For this review, take the finished solid that the model builds, in its own axes (mm). Face numbers are marked on the shaded views. A direction names the side the tool comes from. Coordinates: 2 decimals unless noted, no trailing zeros. Order: outer loops, then holes, each group sorted by start corner. A loop starts at its lowest first (then second) coordinate and runs counter-clockwise, first axis right, second up. Notation, with made-up numbers: (81, 6.5) -> (134, 6.5) arc R32 ccw to (134, 42.5) -> close; hole circle Ø10 at (60, -28). An arc over 180 degrees is marked (long way). Answer as a JSON object with one key per item and string values. Group by question number.
1) Draft analysis for pull direction X (two halves, no side actions). For the marked faces 3, 4, 5 and 6, state which applies: +X half, -X half, draft (parallel to the pull), parting line (faces both ways), or undercut.
2) Add section C-C, the plane x = 56. Write out the cut boundary in (y, z).
3) Add section B-B, the plane z = 26. Write out the cut boundary in (x, y).
4) Machinability: for the marked faces 1 and 2, which of the approach directions +Z, -Z, +X, -X, +Y, -Y give a long, thin tool a straight path to every point of the face, cutting with its end or side? Answer none if there is none.
5) Add section A-A, the plane y = -20.5. Write out the cut boundary in (x, z), then the cut area to 3 significant figures.
6) Wall thickness on L1, parallel to X at y = -50.5, z = 33; L2, parallel to Z at x = 57.5, y = -64.5; L3, parallel to Y at x = 31, z = 45.5: over which ranges is each line inside the solid? List them lowest first.
from build123d import *

# Parameters (mm, degrees)
F1_DEPTH = 76.2
F2_W     = 101.6
F2_H     = 50.8
F3_DEPTH = 50.8


with BuildPart() as f1:
    # F0 (on Front) → F1 (new body)
    with BuildSketch(Plane.XZ):
        Polygon((-68.4001594782, 53.9017294705), (-68.4001594782, -47.6982705295), (83.9998405218, -47.6982705295), (83.9998405218, 53.9017294705), (58.5998405218, 53.9017294705), (58.5998405218, 3.1017294705), (-43.0001594782, 3.1017294705), (-43.0001594782, 53.9017294705), align=None)
    extrude(amount=F1_DEPTH)

    # F2 (on face) → F3 (join)
    with BuildSketch(Plane(origin=(0, 0, 0), x_dir=(-1, 0, 0), z_dir=(0, 1, 0))):
        with Locations((-7.7998405218, 28.5017294705)):
            Rectangle(F2_W, F2_H)
        Polygon((-58.5998405218, 53.9017294705), (-83.9998405218, 53.9017294705), (-83.9998405218, -47.6982705295), (68.4001594782, -47.6982705295), (68.4001594782, 53.9017294705), (43.0001594782, 53.9017294705), (43.0001594782, 3.1017294705), (-58.5998405218, 3.1017294705), align=None)
    extrude(amount=F3_DEPTH)


solid = f1.part
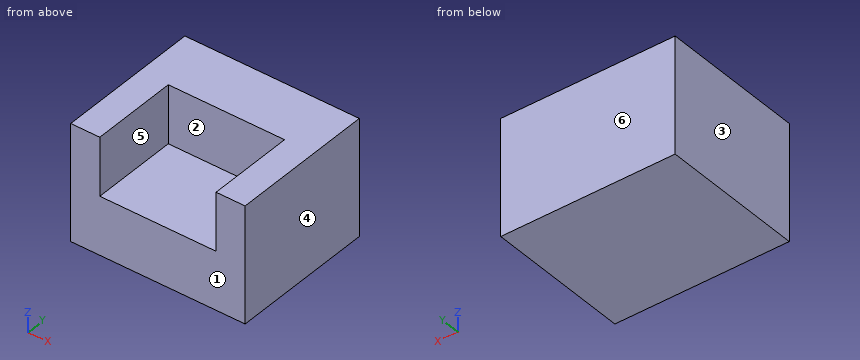
Output values:
{
 "1": {"face 3": "-X half", "face 4": "+X half", "face 5": "undercut", "face 6": "draft"},
 "2": {"outline": "(-76.2, -47.7) -> (50.8, -47.7) -> (50.8, 53.9) -> (0, 53.9) -> (0, 3.1) -> (-76.2, 3.1) -> close"},
 "3": {"outline": "(-68.4, -76.2) -> (-43, -76.2) -> (-43, 0) -> (58.6, 0) -> (58.6, -76.2) -> (84, -76.2) -> (84, 50.8) -> (-68.4, 50.8) -> close"},
 "4": {"face 1": "+Z, -Z, +X, -X, -Y", "face 2": "+Z, -Y"},
 "5": {"outline": "(-68.4, -47.7) -> (84, -47.7) -> (84, 53.9) -> (58.6, 53.9) -> (58.6, 3.1) -> (-43, 3.1) -> (-43, 53.9) -> (-68.4, 53.9) -> close", "area": "10,300 mm²"},
 "6": {"L1": "x = -68.4 to -43, 58.6 to 84", "L2": "z = -47.7 to 3.1", "L3": "y = 0 to 50.8"}
}
